```python
from build123d import *

# Parameters (mm, degrees)
SKETCH1_W           = 35
SKETCH1_H           = 120
SKETCH1_W_2         = 46
SKETCH1_H_2         = 40
BOSS_EXTRUDE1_DEPTH = 7.5
BOSS_EXTRUDE2_DEPTH = 20
SKETCH3_R           = 1.4
CUT_EXTRUDE1_DEPTH  = 5
SKETCH5_R           = 2.95
BOSS_EXTRUDE4_DEPTH = 4
SKETCH6_R           = 1.4
CUT_EXTRUDE2_DEPTH  = 60
SKETCH7_R           = 2.5
CUT_EXTRUDE3_DEPTH  = 10


with BuildPart() as part:
    # Sketch1 → Boss-Extrude1 (new body)
    with BuildSketch(Plane(origin=(0, 0, 0), x_dir=(1, 0, 0), z_dir=(0, 1, 0))):
        with Locations((17.5, 0)):
            Rectangle(SKETCH1_W, SKETCH1_H)
        with Locations((58, 0)):
            Rectangle(SKETCH1_W_2, SKETCH1_H_2)
    extrude(amount=BOSS_EXTRUDE1_DEPTH)

    # Sketch2 → Boss-Extrude2 (add)
    with BuildSketch(Plane(origin=(0, 7.5, 0), x_dir=(1, 0, 0), z_dir=(0, 1, 0))):
        Polygon((35, 2.5), (35, 60), (32.5, 60), (32.5, 27.5), (-35, 27.5), (-35, 25), (32.5, 25), (32.5, -25), (-35, -25), (-35, -27.5), (32.5, -27.5), (32.5, -60), (35, -60), (35, -2.5), (116, -2.5), (116, 2.5), align=None)
    extrude(amount=BOSS_EXTRUDE2_DEPTH)

    # Sketch3 → Cut-Extrude1 (cut)
    with BuildSketch(Plane.XY.offset(2.5)):
        with Locations((111, 25)):
            Circle(SKETCH3_R)
        with Locations((111, 15)):
            Circle(SKETCH3_R)
        with Locations((96, 15)):
            Circle(SKETCH3_R)
        with Locations((96, 25)):
            Circle(SKETCH3_R)
    extrude(amount=-CUT_EXTRUDE1_DEPTH, mode=Mode.SUBTRACT)

    # Sketch5 → Boss-Extrude4 (add)
    with BuildSketch(Plane(origin=(35, 0, 0), x_dir=(0, 0, -1), z_dir=(1, 0, 0))):
        with Locations((-48, 17.5)):
            Circle(SKETCH5_R)
        with Locations(Location((48, 17.5, 0), (0, 0, 180))):
            Circle(SKETCH5_R)
    extrude(amount=BOSS_EXTRUDE4_DEPTH)

    # Sketch6 → Cut-Extrude2 (cut)
    with BuildSketch(Plane.XY.offset(27.5)):
        with Locations((-30, 25)):
            Circle(SKETCH6_R)
        with Locations((-5, 25)):
            Circle(SKETCH6_R)
        with Locations((-30, 15)):
            Circle(SKETCH6_R)
        with Locations((-5, 15)):
            Circle(SKETCH6_R)
    extrude(amount=-CUT_EXTRUDE2_DEPTH, mode=Mode.SUBTRACT)

    # Sketch7 → Cut-Extrude3 (cut)
    with BuildSketch(Plane(origin=(0, 7.5, 0), x_dir=(1, 0, 0), z_dir=(0, 1, 0))):
        with Locations(Location((16.25, 52.5, 0), (0, 0, 270))):
            Circle(SKETCH7_R)
        with Locations(Location((16.25, 35, 0), (0, 0, 270))):
            Circle(SKETCH7_R)
        with Locations(Location((16.25, -35, 0), (0, 0, 270))):
            Circle(SKETCH7_R)
        with Locations(Location((16.25, -52.5, 0), (0, 0, 270))):
            Circle(SKETCH7_R)
    extrude(amount=-CUT_EXTRUDE3_DEPTH, mode=Mode.SUBTRACT)


solid = part.part
```
The listing builds one solid part. Answer for the finished solid, in the listing's coordinates (mm). A direction names the side the tool comes from. Give positions to 0.01 mm unless a question says otherwise; leave off trailing zeros. Write each loop counter-clockwise with the first axis right and the second up, starting at its lowest first coordinate (ties: lowest second). Pieces come first, ordered by that corner, then holes. Notation, with made-up numbers: (49, 41) -> (75, 41) arc R23 cw to (75, 52) -> close; hole circle Ø7 at (33.25, 1.5). An arc over 180 degrees is marked (long way). Write item = value, one per line. Start each with the question number.
1) The part is cut by section C-C, the plane y = 10. Determine the outline of the cut face in (x, z).
2) The part is cut by section D-D, the plane x = -19. Determine the outline of the cut face in (y, z).
3) The part is cut by section B-B, the plane x = 8. Determine the outline of the cut face in (y, z), and give its area (3 significant figures).
4) Determine the mould class of faces 4 (the face through (75, 17, 2.5)), 5 (the face through (15.29, 3.8, -50.19)), 6 (the face through (39, 18, 48)) for opening direction X: +X half, -X half, draft (parallel to the pull), parting line (faces both ways), or undercut.
5) Which of the six approach directions +Z, -Z, +X, -X, +Y, -Y give full straight-line access (tool end or side, diameter ignored) to faces 1 (the face through (36.972, 17.63, 50.947)), 2 (the face through (58, 4, 20)), 3 (the face through (58, 7.5, 11))?
6) The part is cut by section A-A, the plane z = 35. Determine the outline of the cut face in (x, y), and give its area (3 significant figures).
7) Straight lines are drawn through the part: line 1 along Y through (x, z) = (-30, 26.95); line 2 along Z through (x, y) = (1, 16); line 3 along Z through (x, y) = (98.5, 14). For each, find the intervals that lie inside material, in ascending order.
8) Each of these flat-tipped pins is pushed along its axis until it touches: pin 1 (4 mm diameter, centred on x = -1.5, z = 36.5, fed in from +Y); pin 2 (3 mm diameter, centred on y = 19.5, z = -26.5, fed in from +X); pin 3 (3.5 mm diameter, centred on x = -30, y = 25, fed in from -Z). Where does it stop, or does it pass through?
Solutions:
q1.outline = (-35, -27.5) -> (32.5, -27.5) -> (32.5, -60) -> (35, -60) -> (35, -2.5) -> (116, -2.5) -> (116, 2.5) -> (35, 2.5) -> (35, 60) -> (32.5, 60) -> (32.5, 27.5) -> (-35, 27.5) -> (-35, 25) -> (32.5, 25) -> (32.5, -25) -> (-35, -25) -> close
q2.outline = (7.5, -27.5) -> (27.5, -27.5) -> (27.5, -25) -> (7.5, -25) -> close; (7.5, 25) -> (27.5, 25) -> (27.5, 27.5) -> (7.5, 27.5) -> close
q3.outline = (0, -60) -> (7.5, -60) -> (7.5, -27.5) -> (27.5, -27.5) -> (27.5, -25) -> (7.5, -25) -> (7.5, 25) -> (27.5, 25) -> (27.5, 27.5) -> (7.5, 27.5) -> (7.5, 60) -> (0, 60) -> close
q3.area = 1,000 mm²
q4.face_4 = draft
q4.face_5 = undercut
q4.face_6 = +X half
q5.face_1 = +X
q5.face_2 = +Z, +X, +Y, -Y
q5.face_3 = +Z, +X, +Y
q6.outline = (0, 0) -> (13.75, 0) -> (13.75, 7.5) -> (0, 7.5) -> close; (18.75, 0) -> (35, 0) -> (35, 27.5) -> (32.5, 27.5) -> (32.5, 7.5) -> (18.75, 7.5) -> close
q6.area = 275 mm²
q7.line_1 = 7.5 to 13.6, 16.4 to 23.6, 26.4 to 27.5
q7.line_2 = -27.5 to -25, 25 to 27.5
q7.line_3 = -2.5 to 2.5
q8.pin_1 = 7.5
q8.pin_2 = 35
q8.pin_3 = -27.5
